Check sheet for the modelled part. Datum: model origin and axes. Units: mm. Face numbers are marked on the shaded views. A direction names the side the tool comes from. Give positions to 0.01 mm unless a question says otherwise; leave off trailing zeros. Loops run counter-clockwise (first coordinate to the right, second up) from the corner with the lowest first, then second, coordinate; pieces in that order, holes last. Notation, with made-up numbers: M 69.5,34.25 L 82.5,34.25 A12 cw 82.5,45.25 Z; hole C 80,-14.75 d11. An arc over 180 degrees is marked long. Use one line per item in the form item = value.
from build123d import *

# Parameters (mm, degrees)
SKETCH_1_W          = 37.703662968
SKETCH_1_H          = 40
SKETCH_1_R          = 12.5
EXTRUDE_1_DEPTH     = 30
EXTRUDE_3_DEPTH     = 30
SKETCH_9_W          = 21.151556031
SKETCH_9_H          = 33.5604842
CUT_EXTRUDE_5_DEPTH = 30
FILLET_4_R          = 5
CHAMFER_4_SIZE      = 7
FILLET_5_R          = 5
SKETCH_10_R         = 4.000000001
CUT_EXTRUDE_6_DEPTH = 91.362494631
CHAMFER_6_SIZE      = 10
CHAMFER_7_SIZE      = 5


with BuildPart() as part:
    # Эскиз1 → Вытянуть1 (new body)
    with BuildSketch(Plane(origin=(0, 0, 0), x_dir=(1, 0, 0), z_dir=(0, 1, 0))):
        with Locations((-1.148168516, 0)):
            Rectangle(SKETCH_1_W, SKETCH_1_H)
        with Locations(Location((0, 0, 0), (0, 0, 270))):
            Circle(SKETCH_1_R, mode=Mode.SUBTRACT)
    extrude(amount=EXTRUDE_1_DEPTH)

    # Эскиз8 → Вытянуть3 (add)
    with BuildSketch(Plane.XZ):
        Polygon((-20, 20), (-56, -12.013671604), (-56, -42.815306854), (-20, -42.815306854), align=None)
    extrude(amount=-EXTRUDE_3_DEPTH)

    # Эскиз9 → Вырез-Вытянуть5 (cut)
    with BuildSketch(Plane(origin=(0, 0, -42.815306854), x_dir=(-1, 0, 0), z_dir=(0, 0, -1))):
        with Locations((37.872859834, 13.650165161)):
            Rectangle(SKETCH_9_W, SKETCH_9_H)
    extrude(amount=-CUT_EXTRUDE_5_DEPTH, mode=Mode.SUBTRACT)

    # Скругление4
    fillet_4_edges = [part.edges().sort_by_distance(p)[0] for p in [
        (-27.297081818, 15, -12.815306854),
        (-48.448637849, 15, -12.815306854),
    ]]
    fillet(fillet_4_edges, radius=FILLET_4_R)

    # Фаска4
    chamfer_4_edges = [part.edges().sort_by_distance(p)[0] for p in [
        (-52.224318925, 30, -42.815306854),
        (-23.648540909, 30, -42.815306854),
    ]]
    chamfer(chamfer_4_edges, length=CHAMFER_4_SIZE)

    # Скругление5
    fillet_5_edges = [part.edges().sort_by_distance(p)[0] for p in [
        (-20, 15, -20),
    ]]
    fillet(fillet_5_edges, radius=FILLET_5_R)

    # Эскиз10 → Вырез-Вытянуть6 (cut, through all)
    with BuildSketch(Plane.ZY.offset(56)):
        with Locations((-30.109876722, 19.484541516)):
            Circle(SKETCH_10_R)
    extrude(amount=-CUT_EXTRUDE_6_DEPTH, mode=Mode.SUBTRACT)

    # Фаска6
    chamfer_6_edges = [part.edges().sort_by_distance(p)[0] for p in [
        (-23.648540909, 0, -42.815306854),
        (-52.224318925, 0, -42.815306854),
    ]]
    chamfer(chamfer_6_edges, length=CHAMFER_6_SIZE)

    # Фаска7
    chamfer_7_edges = [part.edges().sort_by_distance(p)[0] for p in [
        (17.703662968, 15, -20),
        (17.703662968, 15, 20),
    ]]
    chamfer(chamfer_7_edges, length=CHAMFER_7_SIZE)


solid = part.part
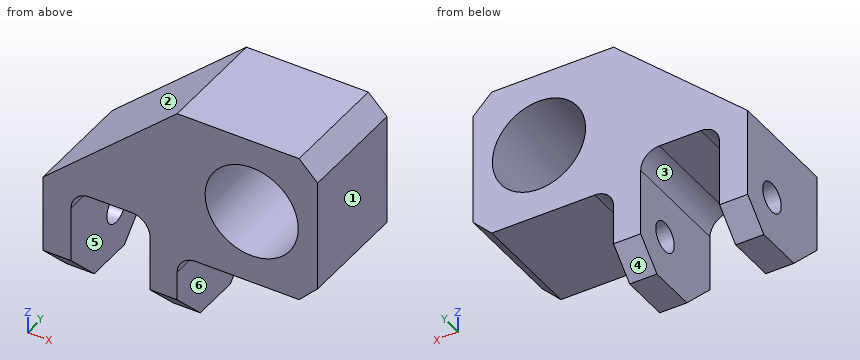
1) Release check for a two-part mould opening along X. For the marked faces 1, 2 and 3 record: pulls with the +X half, pulls with the -X half, needs draft (parallel to the pull), parting line crosses it, or undercut.
Evaluation:
face_1 = pulls with the +X half
face_2 = pulls with the -X half
face_3 = undercut
2) Depth check by flat-ended pin: pin 1 Ø5.5 at (y, z) = (11, -37) entering from +X; pin 2 Ø5 at (x, y) = (-46, 20.5) entering from +Z; pin 3 Ø1.5 at (x, y) = (-47.5, 25) entering from +Z; pin 4 Ø13 at (y, z) = (19.48, -30.11) entering from -X. Enter the tip coordinate at first touch or a pass-through.
Evaluation:
pin_1 = -20
pin_2 = -0.9
pin_3 = -3.79
pin_4 = -56
3) Section check A-A (x = 0). Record the cut outline in (y, z), then the cut area to 3 significant figures.
Evaluation:
outline = M 0,-20 L 30,-20 L 30,-12.5 L 0,-12.5 Z; M 0,12.5 L 30,12.5 L 30,20 L 0,20 Z
area = 450 mm^2
4) Section check B-B (y = 20.5). Record the cut outline in (x, z), then the cut area to 3 significant figures.
Evaluation:
outline = M -56,-42.82 L -48.45,-42.82 L -48.45,-33.98 L -56,-33.98 Z; M -56,-26.24 L -48.45,-26.24 L -48.45,-17.82 A5 cw -43.45,-12.82 L -32.3,-12.82 A5 cw -27.3,-17.82 L -27.3,-26.24 L -20,-26.24 L -20,-25 A5 cw -15,-20 L 12.7,-20 L 17.7,-15 L 17.7,15 L 12.7,20 L -20,20 L -56,-12.01 Z; M -27.3,-42.82 L -20,-42.82 L -20,-33.98 L -27.3,-33.98 Z; hole C 0,0 d25
area = 1,940 mm^2
5) Scan lines: line 1 (X direction, y = 23.5, z = -27); line 2 (Y direction, x = -24, z = -29.5); line 3 (Z direction, x = -15, y = 4). Record each from-to range of solid material in increasing order.
Evaluation:
line_1 = -56 to -48.45, -27.3 to -20
line_2 = 0 to 15.53, 23.44 to 30
line_3 = -20 to 20
6) Section check C-C (z = 5.5). Record the cut outline in (x, y).
Evaluation:
outline = M -36.31,0 L -11.22,0 L -11.22,30 L -36.31,30 Z; M 11.22,0 L 17.7,0 L 17.7,30 L 11.22,30 Z
7) Set-up check for the marked faces 4, 5 and 6: record each of +Z, -Z, +X, -X, +Y, -Y from which the full face is reachable in a straight line by a thin tool's end or side.
Evaluation:
face_4 = -Z, +X, -X, +Y
face_5 = -Z, +Y, -Y
face_6 = -Z, +X, +Y, -Y
8) Section check D-D (y = 5). Record the cut outline in (x, z).
Evaluation:
outline = M -56,-37.82 L -48.45,-37.82 L -48.45,-17.82 A5 cw -43.45,-12.82 L -32.3,-12.82 A5 cw -27.3,-17.82 L -27.3,-37.82 L -20,-37.82 L -20,-25 A5 cw -15,-20 L 12.7,-20 L 17.7,-15 L 17.7,15 L 12.7,20 L -20,20 L -56,-12.01 Z; hole C 0,0 d25
